Read the model definition and answer for the solid it produces. Units are mm, in the model's axes. Face numbers are marked on the shaded views. A direction names the side the tool comes from. Give positions to 0.01 mm unless a question says otherwise; leave off trailing zeros. Order: outer loops, then holes, each group sorted by start corner. A loop starts at its lowest first (then second) coordinate and runs counter-clockwise, first axis right, second up. Notation, with made-up numbers: (33.5, -36) - (66.5, -36) arc R34 cw to (66.5, -4) - close; hole circle Ø11 at (14.5, -22.5). An arc over 180 degrees is marked (long way). Return JSON: item names as keys, results as strings.
```python
from build123d import *

# Parameters (mm, degrees)
F0_R     = 60.575809744
F0_R_2   = 51.7071854394
F0_R_3   = 49.5795397822
F1_DEPTH = 150
F2_R     = 74.8170316814
F3_DEPTH = 25
F4_DEPTH = 10


with BuildPart() as f1:
    # F0 (on Front) → F1 (new body)
    with BuildSketch(Plane.XZ):
        Circle(F0_R)
        Circle(F0_R_2, mode=Mode.SUBTRACT)
        Circle(F0_R_2)
        Circle(F0_R_3, mode=Mode.SUBTRACT)
        Circle(F0_R_3)
        with BuildLine():
            ThreePointArc((47.4934404762, 7.4934404762), (47.9338537115, 3.7582185677), (48.0809581689, 0))
            ThreePointArc((48.0809581689, 0), (47.9338537115, -3.7582185677), (47.4934404762, -7.4934404762))
            ThreePointArc((47.4934404762, -7.4934404762), (33.9983715672, -33.9983715672), (7.4934404762, -47.4934404762))
            ThreePointArc((7.4934404762, -47.4934404762), (0, -48.0809581689), (-7.4934404762, -47.4934404762))
            ThreePointArc((-7.4934404762, -47.4934404762), (-33.9983715672, -33.9983715672), (-47.4934404762, -7.4934404762))
            ThreePointArc((-47.4934404762, -7.4934404762), (-48.0809581689, 0), (-47.4934404762, 7.4934404762))
            ThreePointArc((-47.4934404762, 7.4934404762), (-33.9983715672, 33.9983715672), (-7.4934404762, 47.4934404762))
            ThreePointArc((-7.4934404762, 47.4934404762), (0, 48.0809581689), (7.4934404762, 47.4934404762))
            ThreePointArc((7.4934404762, 47.4934404762), (33.9983715672, 33.9983715672), (47.4934404762, 7.4934404762))
        make_face(mode=Mode.SUBTRACT)
        with BuildLine():
            ThreePointArc((47.4934404762, -7.4934404762), (47.9338537115, -3.7582185677), (48.0809581689, 0))
            ThreePointArc((48.0809581689, 0), (47.9338537115, 3.7582185677), (47.4934404762, 7.4934404762))
            Line((47.4934404762, 7.4934404762), (7.4934404762, 7.4934404762))
            Line((7.4934404762, 7.4934404762), (7.4934404762, 47.4934404762))
            ThreePointArc((7.4934404762, 47.4934404762), (0, 48.0809581689), (-7.4934404762, 47.4934404762))
            Line((-7.4934404762, 47.4934404762), (-7.4934404762, 7.4934404762))
            Line((-7.4934404762, 7.4934404762), (-47.4934404762, 7.4934404762))
            ThreePointArc((-47.4934404762, 7.4934404762), (-48.0809581689, 0), (-47.4934404762, -7.4934404762))
            Line((-47.4934404762, -7.4934404762), (-7.4934404762, -7.4934404762))
            Line((-7.4934404762, -7.4934404762), (-7.4934404762, -47.4934404762))
            ThreePointArc((-7.4934404762, -47.4934404762), (0, -48.0809581689), (7.4934404762, -47.4934404762))
            Line((7.4934404762, -47.4934404762), (7.4934404762, -7.4934404762))
            Line((7.4934404762, -7.4934404762), (47.4934404762, -7.4934404762))
        make_face()
    extrude(amount=F1_DEPTH)

    # F2 (on Front) → F3 (join)
    with BuildSketch(Plane.XZ):
        Circle(F2_R)
    extrude(amount=F3_DEPTH)

    # F4 (cut): faces of the model
    f4_faces = [f1.faces().sort_by_distance(p)[0] for p in [
        (-23.6778496661, -25, 23.6778496661),
        (23.6778496661, -25, 23.6778496661),
        (23.6778496661, -25, -23.6778496661),
        (-23.6778496661, -25, -23.6778496661),
    ]]
    extrude(f4_faces, amount=-F4_DEPTH, mode=Mode.SUBTRACT)


solid = f1.part
```
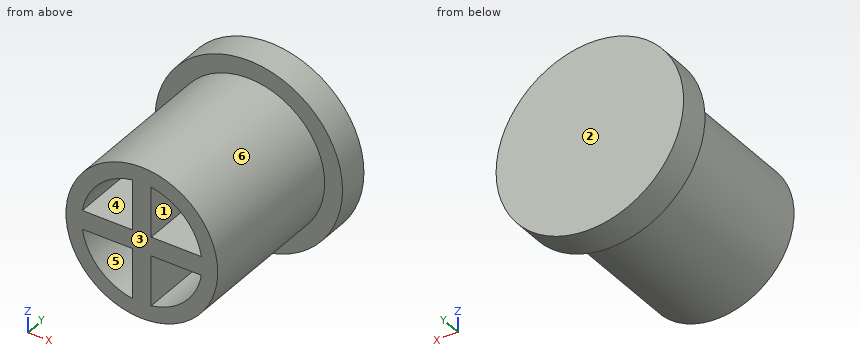
Q1. Determine the mould class of the marked faces 3, 4, 5 and 6 for opening direction X: released by +X, released by -X, zero draft, split by the parting line, or undercut.
Values:
{"face 3": "zero draft", "face 4": "undercut", "face 5": "undercut", "face 6": "split by the parting line"}
Q2. A cutting plane is placed at D-D (z = 20). Write down the section's boundary in (x, y).
Values:
{"outline": "(-72.09, -25) - (-57.18, -25) - (-57.18, -150) - (-43.72, -150) - (-43.72, -15) - (-7.49, -15) - (-7.49, -150) - (7.49, -150) - (7.49, -15) - (43.72, -15) - (43.72, -150) - (57.18, -150) - (57.18, -25) - (72.09, -25) - (72.09, 0) - (-72.09, 0) - close"}
Q3. A cutting plane is placed at C-C (z = 0). Write down the section's boundary in (x, y).
Values:
{"outline": "(-74.82, -25) - (-60.58, -25) - (-60.58, -150) - (60.58, -150) - (60.58, -25) - (74.82, -25) - (74.82, 0) - (-74.82, 0) - close"}
Q4. Consider L1, parallel to X at y = -100, z = 40; L2, parallel to X at y = -90, z = -15.5; L3, parallel to Z at x = -11, y = -53. Determine where each line is inside the solid, lowest interval first.
Values:
{"L1": "x = -45.49 to -26.68, -7.49 to 7.49, 26.68 to 45.49", "L2": "x = -58.56 to -45.51, -7.49 to 7.49, 45.51 to 58.56", "L3": "z = -59.57 to -46.81, -7.49 to 7.49, 46.81 to 59.57"}
Q5. A cutting plane is placed at B-B (x = 0). Write down the section's boundary in (y, z).
Values:
{"outline": "(-150, -60.58) - (-25, -60.58) - (-25, -74.82) - (0, -74.82) - (0, 74.82) - (-25, 74.82) - (-25, 60.58) - (-150, 60.58) - close"}
Q6. Given pin 1 (12 mm diameter, centred on x = 29, y = -73.5, fed in from -Z); pin 2 (2 mm diameter, centred on y = -91, z = 46.5, fed in from +X); pin 3 (5 mm diameter, centred on x = 21.5, y = -40.5, fed in from +Z), each flat-ended and moving along its own axis, determine where each tip first touches the part or whether it passes through.
Values:
{"pin 1": "stops at z = -56.04", "pin 2": "stops at x = 39.99", "pin 3": "stops at z = 57.52"}
Q7. A cutting plane is placed at A-A (y = -59). Write down the section's boundary in (x, z), and give its area (3 significant figures).
Values:
{"outline": "circle Ø121.15 at (0, 0); hole (-47.49, -7.49) arc R48.08 ccw to (-7.49, -47.49) - (-7.49, -7.49) - close; hole (-47.49, 7.49) - (-7.49, 7.49) - (-7.49, 47.49) arc R48.08 ccw to start; hole (7.49, -47.49) arc R48.08 ccw to (47.49, -7.49) - (7.49, -7.49) - close; hole (7.49, 7.49) - (47.49, 7.49) arc R48.08 ccw to (7.49, 47.49) - close", "area": "6,910 mm²"}
Q8. For the marked faces 1 and 2, determine the directions among +Z, -Z, +X, -X, +Y, -Y from which every point of the face is accessible in a straight line to the end or side of a thin tool.
Values:
{"face 1": "-Y", "face 2": "+Z, -Z, +X, -X, +Y"}
